Model file for the job. Use its own axes, mm. Face numbers are marked on the shaded views. A direction names the side the tool comes from. Round coordinates to 2 decimals unless told otherwise and drop trailing zeros. Write each loop counter-clockwise with the first axis right and the second up, starting at its lowest first coordinate (ties: lowest second). Pieces come first, ordered by that corner, then holes. Notation, with made-up numbers: (23, -19.75) - (46, -19.75) arc R7 cw to (46, -11.75) - close; hole circle Ø1 at (27.5, 19.25). An arc over 180 degrees is marked (long way). Answer as a JSON object with one key per item and string values. Group by question number.
from build123d import *

# Parameters (mm, degrees)
ESBO_O3_W             = 8
ESBO_O3_H             = 8
CORTE_EXTRUS_O1_DEPTH = 20
CHANFRO1_SIZE         = 2


with BuildPart() as part:
    # Sketch1 → Revolve1 (revolve)
    with BuildSketch(Plane.XY):
        Polygon((0, 150), (12.5, 150), (12.5, 5), (15, 5), (15, 0), (0, 0), align=None)
    revolve(axis=Axis((0, 0, 0), (0, 1, 0)))

    # Esboço3 → Corte-extrusão1 (cut)
    with BuildSketch(Plane(origin=(0, 150, 0), x_dir=(1, 0, 0), z_dir=(0, 1, 0))):
        with Locations((-11, 0)):
            Rectangle(ESBO_O3_W, ESBO_O3_H)
    extrude(amount=-CORTE_EXTRUS_O1_DEPTH, mode=Mode.SUBTRACT)

    # Chanfro1
    chanfro1_edges = [part.edges().sort_by_distance(p)[0] for p in [
        (2.026821276, 150, -12.33458534),
    ]]
    chamfer(chanfro1_edges, length=CHANFRO1_SIZE)


solid = part.part
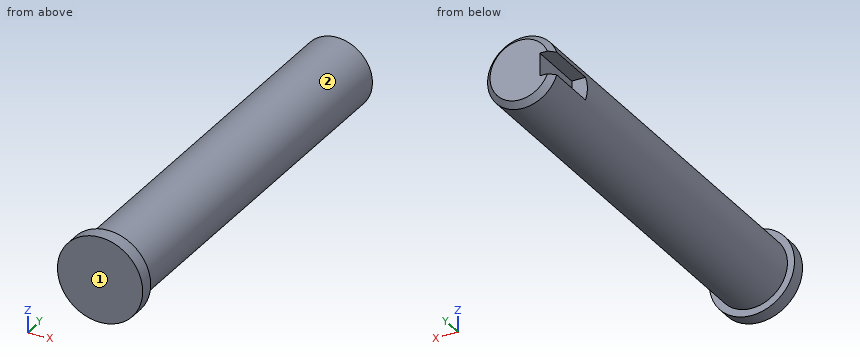
(1) Slice it at B-B (z = 0). Write the cut outline in (x, y).
(2) Drill centre lines: line 1 (Y direction, x = -8.5, z = 11.25); line 2 (X direction, y = 116, z = 0.25); line 3 (X direction, y = 132, z = 0.5). Where is each one in solid material? Low to high. Write a range as from..to.
(3) Slice it at A-A (x = 0). Write the cut outline in (y, z).
(4) 3-axis set-ups, long thin cutter, end or side, ignore diameter. For the marked faces 1 and 2: which of +Z, -Z, +X, -X, +Y, -Y reach the whole face in a straight line?
(5) Slice it at C-C (y = 72). Write the cut outline in (x, z), then the cut area to 3 significant figures.
(6) Flat gauge pins, fed straight in: pin 1 (2.5 mm diameter, centred on x = -9.5, y = 143, fed in from -Z); pin 2 (1.6 mm diameter, centred on x = -9, z = 0.5, fed in from +Y); pin 3 (2 mm diameter, centred on x = -6, y = 90.5, fed in from +Z); pin 4 (8 mm diameter, centred on x = -6.5, z = 4, fed in from -Y). Where does each tip first touch, or does it go through?
Answer:
{
 "1": {"outline": "(-15, 0) - (15, 0) - (15, 5) - (12.5, 5) - (12.5, 148) - (10.5, 150) - (-7, 150) - (-7, 130) - (-12.5, 130) - (-12.5, 5) - (-15, 5) - close"},
 "2": {"line 1": "0..5", "line 2": "-12.5..12.5", "line 3": "-7..12.49"},
 "3": {"outline": "(0, -15) - (5, -15) - (5, -12.5) - (148, -12.5) - (150, -10.5) - (150, 10.5) - (148, 12.5) - (5, 12.5) - (5, 15) - (0, 15) - close"},
 "4": {"face 1": "+Z, -Z, +X, -X, -Y", "face 2": "+Y"},
 "5": {"outline": "circle Ø25 at (0, 0)", "area": "491 mm²"},
 "6": {"pin 1": "z = -9.39", "pin 2": "y = 130", "pin 3": "z = 11.46", "pin 4": "y = 0"}
}
